from build123d import *

# Parameters (mm, degrees)
SKETCH2_W           = 6.18
SKETCH2_H           = 3.2
BOSS_EXTRUDE1_DEPTH = 2
BOSS_EXTRUDE2_DEPTH = 1.87
SKETCH4_R           = 4.75
SKETCH4_R_2         = 3
BOSS_EXTRUDE3_DEPTH = 4
FILLET1_R           = 2


with BuildPart() as part:
    # Sketch1 → Revolve1 (revolve)
    with BuildSketch(Plane.XY):
        with BuildLine():
            Line((5.25, 36.6), (5.25, 19.5))
            Line((5.25, 19.5), (2.034602195, 1.7))
            ThreePointArc((2.034602195, 1.7), (1.325670217, 0.480936184), (0, 0))
            Line((0, 0), (0, 38.6))
            Line((0, 38.6), (6.35, 38.6))
            Line((6.35, 38.6), (6.35, 36.6))
            Line((6.35, 36.6), (5.25, 36.6))
        make_face()
    revolve(axis=Axis((0, 0, 0), (0, 1, 0)))

    # Sketch2 → Boss-Extrude1 (add)
    with BuildSketch(Plane(origin=(0, 38.6, 0), x_dir=(1, 0, 0), z_dir=(0, 1, 0))):
        with Locations((0, 7.147467891)):
            Rectangle(SKETCH2_W, SKETCH2_H)
    extrude(amount=-BOSS_EXTRUDE1_DEPTH)

    # Sketch3 → Boss-Extrude2 (add)
    with BuildSketch(Plane(origin=(0, 0, -8.747467891), x_dir=(-1, 0, 0), z_dir=(0, 0, -1))):
        with BuildLine():
            Line((-2.9, 18.8), (2.9, 18.8))
            Line((2.9, 18.8), (5.931288007, 26.449633522))
            ThreePointArc((5.931288007, 26.449633522), (6.37843004, 28.941528165), (5.821199394, 31.411137227))
            Line((5.821199394, 31.411137227), (3.09, 37.5))
            Line((3.09, 37.5), (3.09, 38.6))
            Line((3.09, 38.6), (-3.09, 38.6))
            Line((-3.09, 38.6), (-3.09, 37.5))
            Line((-3.09, 37.5), (-5.821199394, 31.411137227))
            ThreePointArc((-5.821199394, 31.411137227), (-6.37843004, 28.941528165), (-5.931288007, 26.449633522))
            Line((-5.931288007, 26.449633522), (-2.9, 18.8))
        make_face()
    extrude(amount=BOSS_EXTRUDE2_DEPTH)

    # Sketch4 → Boss-Extrude3 (add)
    with BuildSketch(Plane(origin=(0, 0, -10.617467891), x_dir=(-1, 0, 0), z_dir=(0, 0, -1))):
        with Locations((0, 28.8)):
            Circle(SKETCH4_R)
        with Locations((0, 28.8)):
            Circle(SKETCH4_R_2, mode=Mode.SUBTRACT)
    extrude(amount=BOSS_EXTRUDE3_DEPTH)

    # Fillet1
    fillet1_edges = [part.edges().sort_by_distance(p)[0] for p in [
        (0, 38.6, -10.617467891),
    ]]
    fillet(fillet1_edges, radius=FILLET1_R)


solid = part.part
Source: CAD feature listing. Evaluate the final solid. Frame: model axes, mm. A direction names the side the tool comes from. Coordinates: 2 decimals unless noted, no trailing zeros. Order: outer loops, then holes, each group sorted by start corner. A loop starts at its lowest first (then second) coordinate and runs counter-clockwise, first axis right, second up.
Item 1: Cut plane D-D (z = -8.25). Return loops of the section in (x, y).
Output values:
outline: (-3.09, 36.6) - (3.09, 36.6) - (3.09, 38.6) - (-3.09, 38.6) - close
Item 2: Cut plane C-C (x = 0). Return loops of the section in (y, z), plus the area to 3 significant figures.
Output values:
outline: (1.7, -2.03) - (19.5, -5.25) - (36.6, -5.25) - (36.6, -8.75) - (18.8, -8.75) - (18.8, -10.62) - (24.05, -10.62) - (24.05, -14.62) - (25.8, -14.62) - (25.8, -10.62) - (31.8, -10.62) - (31.8, -14.62) - (33.55, -14.62) - (33.55, -10.62) - (36.6, -10.62) arc R2 ccw to (38.6, -8.62) - (38.6, 6.35) - (36.6, 6.35) - (36.6, 5.25) - (19.5, 5.25) - (1.7, 2.03) arc R2.07 ccw to start
area: 395 mm2
Item 3: Cut plane A-A (y = 28.8). Return loops of the section in (x, z), plus the area to 3 significant figures.
Output values:
outline: (-6.38, -10.62) - (-4.75, -10.62) - (-4.75, -14.62) - (-3, -14.62) - (-3, -10.62) - (3, -10.62) - (3, -14.62) - (4.75, -14.62) - (4.75, -10.62) - (6.38, -10.62) - (6.38, -8.75) - (-6.38, -8.75) - close; circle Ø10.5 at (0, 0)
area: 124 mm2
Item 4: First-contact query: P1, Ø6, axis at x = -4, y = 20.5, coming from the +Z side; P2, Ø5, axis at x = 4, y = 15, coming from the -Z side; P3, Ø1.5, axis at x = -0.5, y = 18.5, coming from the -Z side. Flat tips, straight axial feed; report the tip coordinate or a pass-through.
Output values:
P1: stops at z = 5.15
P2: stops at z = -4.29
P3: stops at z = -10.62
Item 5: Material intervals for line 1 (Y direction, x = 0, z = -12.6); line 2 (Y direction, x = 0.25, z = -7.75); line 3 (Z direction, x = 2, y = 30.5), sorted ascending.
Output values:
line 1: y = 24.05 to 25.8, 31.8 to 33.55
line 2: y = 36.6 to 38.6
line 3: z = -10.62 to -8.75, -4.85 to 4.85
Item 6: Set-up query: faces 1 (the face through (-2.192, 24.586, -12.589)), 2 (the face through (-3.09, 38, -7)), 3 (the face through (-4.475, 34.413, -9.669)), 4 (the face through (4.437, 22.678, -9.669)). Return all of +Z, -Z, +X, -X, +Y, -Y with unobstructed straight access to the full face (end or side cutting, diameter ignored); none if empty.
Output values:
face 1: -Z
face 2: -X, +Y
face 3: -Z, -X, +Y
face 4: -Z, +X, -Y
Item 7: Cut plane B-B (z = 0). Return loops of the section in (x, y).
Output values:
outline: (-6.35, 36.6) - (-5.25, 36.6) - (-5.25, 19.5) - (-2.03, 1.7) arc R2.07 ccw to (2.03, 1.7) - (5.25, 19.5) - (5.25, 36.6) - (6.35, 36.6) - (6.35, 38.6) - (-6.35, 38.6) - close
Item 8: Pull-direction query (X, two-part tool) for faces 5 (the face through (0, 29, -10.617)), 6 (the face through (0, 18.8, -10)), 7 (the face through (3.09, 38, -7)); classes: pulls with the +X half, pulls with the -X half, needs draft (parallel to the pull), parting line crosses it, or undercut.
Output values:
face 5: undercut
face 6: needs draft
face 7: pulls with the +X half
